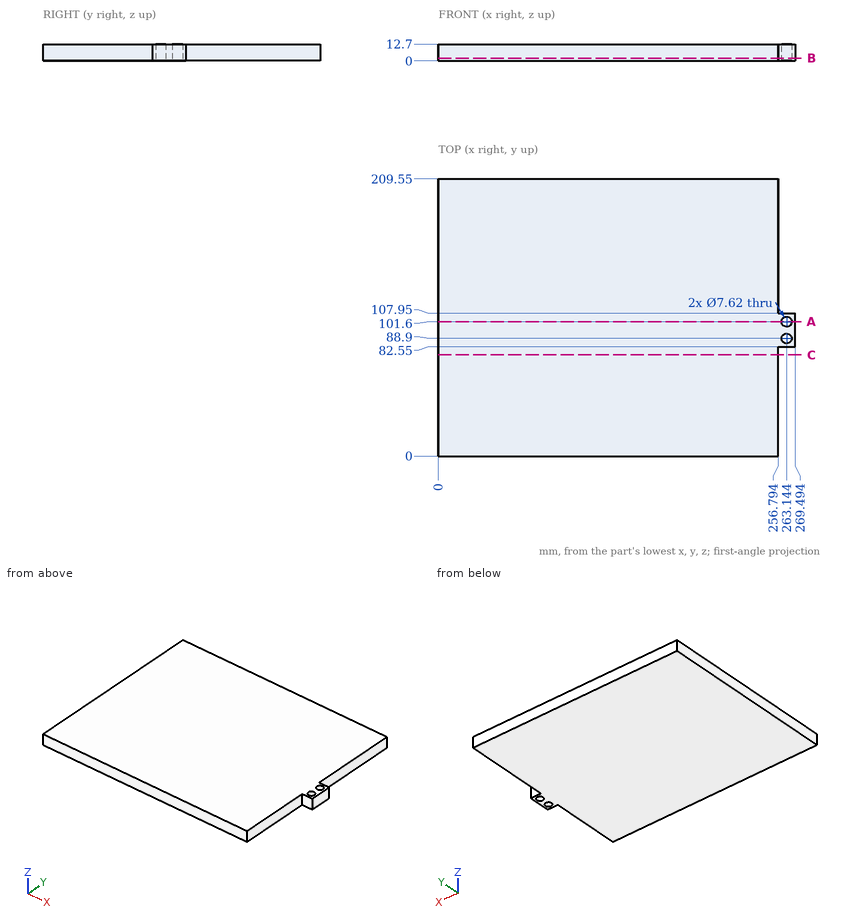
Here's the drawing with two shaded views (mm, measured from the low corner). I have some questions. Coordinates: 2 decimals unless noted, no trailing zeros. Write each loop counter-clockwise with the first axis right and the second up, starting at its lowest first coordinate (ties: lowest second). Pieces come first, ordered by that corner, then holes. Notation, with made-up numbers: M 75,-32 L 99,-32 A13 cw 99,-13 Z; hole C -33.75,64.25 d2. An arc over 180 degrees is marked long. Answer as CSV lines item,"result".
Item 1: Imagine slicing it at A-A on y = 101.6. List the corners of the cut face in (x, z) for me.
Geometry results:
outline,"M 0,0 L 259.33,0 L 259.33,12.7 L 0,12.7 Z; M 266.95,0 L 269.49,0 L 269.49,12.7 L 266.95,12.7 Z"
Item 2: Imagine slicing it at B-B on z = 2. List the corners of the cut face in (x, y) for me.
Geometry results:
outline,"M 0,0 L 256.79,0 L 256.79,82.55 L 269.49,82.55 L 269.49,107.95 L 256.79,107.95 L 256.79,209.55 L 0,209.55 Z; hole C 263.14,88.9 d7.62; hole C 263.14,101.6 d7.62"
Item 3: Imagine slicing it at C-C on y = 76.5. List the corners of the cut face in (x, z) for me, plus the area to 3 significant figures.
Geometry results:
outline,"M 0,0 L 256.79,0 L 256.79,12.7 L 0,12.7 Z"
area,"3,260 mm2"
Item 4: Please list where these lines run through material, in increasing order: line 1 along X through (y, z) = (35, 8.75); line 2 along X through (y, z) = (89.5, 12.25).
Geometry results:
line 1,"x = 0 to 256.79"
line 2,"x = 0 to 259.38, 266.91 to 269.49"
Item 5: I'm going to push a flat-ended pin straight in: P1, Ø4, axis at y = 35.5, z = 8, coming from the +X side. Where does the tip first touch, or does it pass through?
Geometry results:
P1,"stops at x = 256.79"
